```python
from build123d import *

# Parameters (mm, degrees)
SKETCH1_W           = 57
SKETCH1_H           = 8
BOSS_EXTRUDE1_DEPTH = 2.85
CUT_EXTRUDE1_DEPTH  = 29.920105463
SKETCH3_R           = 1.5
CUT_EXTRUDE2_DEPTH  = 29.920105463


with BuildPart() as part:
    # Sketch1 → Boss-Extrude1 (new body)
    with BuildSketch(Plane.XY):
        Rectangle(SKETCH1_W, SKETCH1_H)
    extrude(amount=BOSS_EXTRUDE1_DEPTH)

    # Sketch2 → Cut-Extrude1 (cut, through all)
    with BuildSketch(Plane.XY.offset(2.85)):
        with BuildLine():
            Line((24.5, -4), (29.5, -4))
            Line((29.5, -4), (29.5, 4))
            Line((29.5, 4), (24.5, 4))
            ThreePointArc((24.5, 4), (28.5, 0), (24.5, -4))
        make_face()
    cut_extrude1 = extrude(amount=-CUT_EXTRUDE1_DEPTH, mode=Mode.SUBTRACT)

    # Sketch3 → Cut-Extrude2 (cut, through all)
    with BuildSketch(Plane.XY.offset(2.85)):
        with Locations((24.5, 0)):
            Circle(SKETCH3_R)
    cut_extrude2 = extrude(amount=-CUT_EXTRUDE2_DEPTH, mode=Mode.SUBTRACT)

    # Mirror1: Cut-Extrude1, Cut-Extrude2 across plane
    add(cut_extrude1.mirror(Plane(origin=(0, 0, 0), x_dir=(0, 0, 1), z_dir=(1, 0, 0))), mode=Mode.SUBTRACT)
    add(cut_extrude2.mirror(Plane(origin=(0, 0, 0), x_dir=(0, 0, 1), z_dir=(1, 0, 0))), mode=Mode.SUBTRACT)


solid = part.part
```
Here's how the part is built. I have some questions about the finished solid (model axes, mm). Give positions to 0.01 mm unless a question says otherwise; leave off trailing zeros. Order: outer loops, then holes, each group sorted by start corner. A loop starts at its lowest first (then second) coordinate and runs counter-clockwise, first axis right, second up. Notation, with made-up numbers: M -11.75,28 L 12.25,28 A34 cw 12.25,66 Z; hole C 49.25,42 d1. An arc over 180 degrees is marked long. Use a Markdown table: item, result. Add a question column.
1. If we mould it in two halves opening along Y, with no side actions, what happens to faces 1 (the cylindrical face through (28.5, 0.1, 1.4)), 2 (the flat face through (0, 0, 0)), 3 (the cylindrical face through (-23, 0, 1))? For each: +Y half, -Y half, draft (parallel to the pull), parting line (faces both ways), or undercut.
2. Suppose I cut it at C-C (y = 3). List the corners of the cut face in (x, z) for me, and give its area (3 significant figures).
3. Suppose I cut it at A-A (y = 0). List the corners of the cut face in (x, z) for me.
4. Suppose I cut it at B-B (z = 0.8). List the corners of the cut face in (x, y) for me, and give its area (3 significant figures).
5. I need wall thicknesses on probe 1 along X at (y, z) = (1.25, 2.05); probe 2 along Y at (x, z) = (24.5, 1.25); probe 3 along X at (y, z) = (-1, 2.05). Which ranges of each line are inside material? Lowest first, please. Write a range as from..to.
6. For pin 1 Ø1 at (y, z) = (2, 1) entering from -X, with a flat end and sliding along its axis, tell me the tip position at first contact or that it passes through.
Results list:
| question | item | result |
|---|---|---|
| 1 | face 1 | parting line |
| 1 | face 2 | draft |
| 1 | face 3 | undercut |
| 2 | outline | M -27.15,0 L 27.15,0 L 27.15,2.85 L -27.15,2.85 Z |
| 2 | area | 155 mm² |
| 3 | outline | M -28.5,0 L -26,0 L -26,2.85 L -28.5,2.85 Z; M -23,0 L 23,0 L 23,2.85 L -23,2.85 Z; M 26,0 L 28.5,0 L 28.5,2.85 L 26,2.85 Z |
| 4 | outline | M -24.5,-4 L 24.5,-4 A4 ccw 24.5,4 L -24.5,4 A4 ccw Z; hole C -24.5,0 d3; hole C 24.5,0 d3 |
| 4 | area | 428 mm² |
| 5 | probe 1 | x = -28.3..-25.33, -23.67..23.67, 25.33..28.3 |
| 5 | probe 2 | y = -4..-1.5, 1.5..4 |
| 5 | probe 3 | x = -28.37..-25.62, -23.38..23.38, 25.62..28.37 |
| 6 | pin 1 | stops at x = -28.21 |
